For this review, take the finished solid that the model builds, in its own axes (mm). Face numbers are marked on the shaded views. A direction names the side the tool comes from. Round coordinates to 2 decimals unless told otherwise and drop trailing zeros. Order: outer loops, then holes, each group sorted by start corner. A loop starts at its lowest first (then second) coordinate and runs counter-clockwise, first axis right, second up. Notation, with made-up numbers: (30, -7.5) - (54, -7.5) arc R18 cw to (54, 7.5) - close; hole circle Ø3 at (66.25, -32). An arc over 180 degrees is marked (long way). One line per item, written item: value.
```python
from build123d import *

# Parameters (mm, degrees)
F0_W     = 64.647466
F0_H     = 2.486437
F1_DEPTH = 120
F2_W     = 112.995804
F2_H     = 127.987776
F3_DEPTH = 10
F4_W     = 57.398408
F4_H     = 25.908977
F5_DEPTH = 25


with BuildPart() as f1:
    # F0 (on Front) → F1 (new body)
    with BuildSketch(Plane.XZ):
        with Locations((0, 57.010516)):
            Rectangle(F0_W, F0_H)
    extrude(amount=F1_DEPTH)

    # F2 (on Front) → F3 (join)
    with BuildSketch(Plane.XZ):
        with Locations((0, 17.450197)):
            Rectangle(F2_W, F2_H)
    extrude(amount=F3_DEPTH)

    # F4 (on face) → F5 (cut)
    with BuildSketch(Plane(origin=(0, 0, 0), x_dir=(-1, 0, 0), z_dir=(0, 1, 0))):
        with Locations((0, -18.103005)):
            Rectangle(F4_W, F4_H)
    extrude(amount=-F5_DEPTH, mode=Mode.SUBTRACT)


solid = f1.part
```
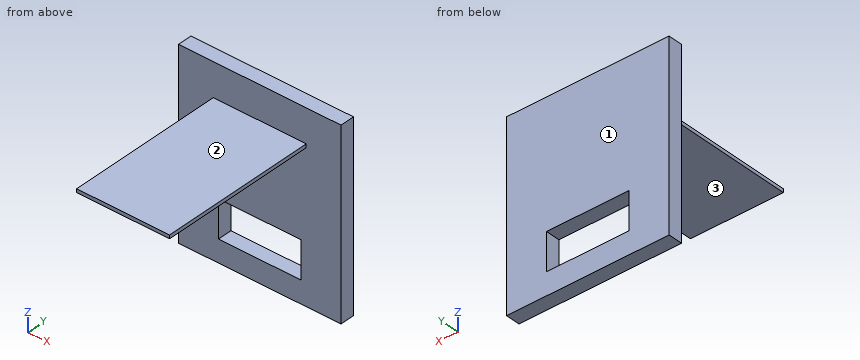
Item 1: Take a section at B-B (x = -27). Write out the cut boundary in (y, z).
Returned:
outline: (-120, 55.77) - (-10, 55.77) - (-10, -5.15) - (0, -5.15) - (0, 81.44) - (-10, 81.44) - (-10, 58.25) - (-120, 58.25) - close; (-10, -46.54) - (0, -46.54) - (0, -31.06) - (-10, -31.06) - close
Item 2: Take a section at D-D (y = -83). Write out the cut boundary in (x, z).
Returned:
outline: (-32.32, 55.77) - (32.32, 55.77) - (32.32, 58.25) - (-32.32, 58.25) - close
Item 3: Machinability: for the marked faces 1, 2 and 3, which of the approach directions +Z, -Z, +X, -X, +Y, -Y give a long, thin tool a straight path to every point of the face, cutting with its end or side? Answer none if there is none.
Returned:
face 1: +Z, -Z, +X, -X, +Y
face 2: +Z, +X, -X, -Y
face 3: -Z, +X, -X, -Y
Item 4: Take a section at A-A (z = -16.5). Write out the cut boundary in (x, y), plus the area to 3 significant figures.
Returned:
outline: (-56.5, -10) - (-28.7, -10) - (-28.7, 0) - (-56.5, 0) - close; (28.7, -10) - (56.5, -10) - (56.5, 0) - (28.7, 0) - close
area: 556 mm^2
Item 5: Take a section at C-C (z = 28.5). Write out the cut boundary in (x, y).
Returned:
outline: (-56.5, -10) - (56.5, -10) - (56.5, 0) - (-56.5, 0) - close
Item 6: Wall thickness on line 1 (Z direction, x = -6, y = -6.5); line 2 (Y direction, x = -49.5, z = 60.5); line 3 (Z direction, x = -4, y = -45): over which ranges is each line inside the solid? List them lowest first.
Returned:
line 1: -46.54 to -31.06, -5.15 to 81.44
line 2: -10 to 0
line 3: 55.77 to 58.25
Item 7: For P1, Ø5, axis at x = -15.5, y = -72, coming from the -Z side; P2, Ø1.5, axis at x = -17, y = -106, coming from the +Z side; P3, Ø2, axis at y = -40.5, z = 57.5, coming from the +X side, all flat-tipped, find the tip position at first contact; note any pin that passes through.
Returned:
P1: z = 55.77
P2: z = 58.25
P3: x = 32.32
